from build123d import *

# Parameters (mm, degrees)
BOSS_EXTRUDE1_DEPTH = 5.07492
SKETCH6_R           = 22.225
BOSS_EXTRUDE3_DEPTH = 5.07492
SKETCH2_3_R         = 6.35
CUT_EXTRUDE2_DEPTH  = 5.588
SKETCH8_W           = 2.728150378
SKETCH8_H           = 127
BOSS_EXTRUDE4_DEPTH = 5.07492
SKETCH9_W           = 1.905
SKETCH9_H           = 127
BOSS_EXTRUDE5_DEPTH = 5.07492
SKETCH12_R          = 3
CUT_EXTRUDE3_DEPTH  = 400.05
CUT_EXTRUDE4_START  = -5.07492
SKETCH13_R          = 22.86
SKETCH13_R_2        = 2
SKETCH13_R_3        = 6.35
CUT_EXTRUDE4_DEPTH  = 0.254
CUT_EXTRUDE6_START  = -127
SKETCH13_2_R        = 2
CUT_EXTRUDE6_DEPTH  = 127
SKETCH17_R          = 2.9972
CUT_EXTRUDE7_DEPTH  = 152.4
CUT_EXTRUDE8_START  = -1549.4
SKETCH13_3_R        = 6.35
CUT_EXTRUDE8_DEPTH  = 1549.4
SKETCH18_R          = 3.175
SKETCH18_R_2        = 2.159
SKETCH18_R_3        = 1.524
CUT_EXTRUDE9_DEPTH  = 6.35
SKETCH19_R          = 1.905
CUT_EXTRUDE10_DEPTH = 6.35


with BuildPart() as part:
    # Sketch2 → Boss-Extrude1 (new body)
    with BuildSketch(Plane.XY):
        with BuildLine():
            Line((-143.383, -31.75), (-127.127, -31.75))
            ThreePointArc((-127.127, -31.75), (-123.317, -30.48), (-119.507, -31.75))
            Line((-119.507, -31.75), (119.253, -31.75))
            ThreePointArc((119.253, -31.75), (123.063, -30.48), (126.873, -31.75))
            Line((126.873, -31.75), (143.383, -31.75))
            Line((143.383, -31.75), (143.383, 95.25))
            Line((143.383, 95.25), (-143.383, 95.25))
            Line((-143.383, 95.25), (-143.383, -31.75))
        make_face()
    extrude(amount=-BOSS_EXTRUDE1_DEPTH)

    # Sketch6 → Boss-Extrude3 (add)
    with BuildSketch(Plane(origin=(0, 0, -5.07492), x_dir=(-1, 0, 0), z_dir=(0, 0, -1))):
        with Locations((-123.063, -36.83)):
            Circle(SKETCH6_R)
        with Locations((123.317, -36.83)):
            Circle(SKETCH6_R)
    extrude(amount=-BOSS_EXTRUDE3_DEPTH)

    # Sketch2<3> → Cut-Extrude2 (cut)
    with BuildSketch(Plane.XY):
        with Locations((-123.317, -36.83)):
            Circle(SKETCH2_3_R)
        with Locations((123.063, -36.83)):
            Circle(SKETCH2_3_R)
    extrude(amount=-CUT_EXTRUDE2_DEPTH, mode=Mode.SUBTRACT)

    # Sketch8 → Boss-Extrude4 (add)
    with BuildSketch(Plane(origin=(0, 0, -5.07492), x_dir=(-1, 0, 0), z_dir=(0, 0, -1))):
        with Locations((144.139824811, 31.75)):
            Rectangle(SKETCH8_W, SKETCH8_H)
    extrude(amount=-BOSS_EXTRUDE4_DEPTH)

    # Sketch9 → Boss-Extrude5 (add)
    with BuildSketch(Plane(origin=(0, 0, -5.07492), x_dir=(-1, 0, 0), z_dir=(0, 0, -1))):
        with Locations((-144.3355, 31.75)):
            Rectangle(SKETCH9_W, SKETCH9_H)
    extrude(amount=-BOSS_EXTRUDE5_DEPTH)

    # Sketch12 → Cut-Extrude3 (cut)
    with BuildSketch(Plane.XY):
        with Locations((-123.317, 76.2)):
            Circle(SKETCH12_R)
        with Locations((123.063, 76.2)):
            Circle(SKETCH12_R)
    extrude(amount=-CUT_EXTRUDE3_DEPTH, mode=Mode.SUBTRACT)

    # Sketch13 → Cut-Extrude4 (cut)
    # profile 1 of 2: a face of its own
    with BuildSketch(Plane(origin=(0, 0, -5.07492), x_dir=(-1, 0, 0), z_dir=(0, 0, -1)).offset(CUT_EXTRUDE4_START)):
        with Locations(Location((23.352511843, 49.53, 0), (0, 0, 180))):
            Circle(SKETCH13_R)
        with Locations(Location((23.352511843, 67.0306, 0), (0, 0, 180))):
            Circle(SKETCH13_R_2, mode=Mode.SUBTRACT)
        with Locations(Location((40.853111843, 49.53, 0), (0, 0, 180))):
            Circle(SKETCH13_R_2, mode=Mode.SUBTRACT)
        with Locations(Location((23.352511843, 32.0294, 0), (0, 0, 180))):
            Circle(SKETCH13_R_2, mode=Mode.SUBTRACT)
        with Locations(Location((5.851911843, 49.53, 0), (0, 0, 180))):
            Circle(SKETCH13_R_2, mode=Mode.SUBTRACT)
        with Locations(Location((23.352511843, 49.53, 0), (0, 0, 180))):
            Circle(SKETCH13_R_3, mode=Mode.SUBTRACT)
    # profile 2 of 2: a face of its own
    with BuildSketch(Plane(origin=(0, 0, -5.07492), x_dir=(-1, 0, 0), z_dir=(0, 0, -1)).offset(CUT_EXTRUDE4_START)):
        with Locations(Location((-32.2961, 1.27, 0), (0, 0, 180))):
            Circle(SKETCH13_R)
        with Locations(Location((-32.2961, 18.7706, 0), (0, 0, 180))):
            Circle(SKETCH13_R_2, mode=Mode.SUBTRACT)
        with Locations(Location((-14.7955, 1.27, 0), (0, 0, 180))):
            Circle(SKETCH13_R_2, mode=Mode.SUBTRACT)
        with Locations(Location((-32.2961, -16.2306, 0), (0, 0, 180))):
            Circle(SKETCH13_R_2, mode=Mode.SUBTRACT)
        with Locations(Location((-49.7967, 1.27, 0), (0, 0, 180))):
            Circle(SKETCH13_R_2, mode=Mode.SUBTRACT)
        with Locations(Location((-32.2961, 1.27, 0), (0, 0, 180))):
            Circle(SKETCH13_R_3, mode=Mode.SUBTRACT)
    extrude(amount=CUT_EXTRUDE4_DEPTH, mode=Mode.SUBTRACT)

    # Sketch13<2> → Cut-Extrude6 (cut)
    with BuildSketch(Plane(origin=(0, 0, -5.07492), x_dir=(-1, 0, 0), z_dir=(0, 0, -1)).offset(CUT_EXTRUDE6_START)):
        with Locations((-32.2961, 18.7706)):
            Circle(SKETCH13_2_R)
        with Locations((-49.7967, 1.27)):
            Circle(SKETCH13_2_R)
        with Locations((-14.7955, 1.27)):
            Circle(SKETCH13_2_R)
        with Locations((-32.2961, -16.2306)):
            Circle(SKETCH13_2_R)
        with Locations((23.352511843, 32.0294)):
            Circle(SKETCH13_2_R)
        with Locations((23.352511843, 67.0306)):
            Circle(SKETCH13_2_R)
        with Locations((40.853111843, 49.53)):
            Circle(SKETCH13_2_R)
        with Locations((5.851911843, 49.53)):
            Circle(SKETCH13_2_R)
    extrude(amount=CUT_EXTRUDE6_DEPTH, mode=Mode.SUBTRACT)

    # Sketch17 → Cut-Extrude7 (cut)
    with BuildSketch(Plane(origin=(0, 0, -5.07492), x_dir=(-1, 0, 0), z_dir=(0, 0, -1))):
        with Locations((87.0839, -19.05)):
            Circle(SKETCH17_R)
        with Locations((-86.868, -16.51)):
            Circle(SKETCH17_R)
    extrude(amount=-CUT_EXTRUDE7_DEPTH, mode=Mode.SUBTRACT)

    # Sketch13<3> → Cut-Extrude8 (cut)
    with BuildSketch(Plane(origin=(0, 0, -5.07492), x_dir=(-1, 0, 0), z_dir=(0, 0, -1)).offset(CUT_EXTRUDE8_START)):
        with Locations((-32.2961, 1.27)):
            Circle(SKETCH13_3_R)
        with Locations((23.352511843, 49.53)):
            Circle(SKETCH13_3_R)
    extrude(amount=CUT_EXTRUDE8_DEPTH, mode=Mode.SUBTRACT)

    # Sketch18 → Cut-Extrude9 (cut)
    with BuildSketch(Plane(origin=(0, 0, -5.07492), x_dir=(-1, 0, 0), z_dir=(0, 0, -1))):
        with Locations((14.5669, -22.225)):
            Circle(SKETCH18_R)
        with Locations((-68.691950102, 24.511)):
            Circle(SKETCH18_R_2)
        with Locations((-62.682085042, -3.620822534)):
            Circle(SKETCH18_R_3)
        with Locations((-1.953743286, -3.620822534)):
            Circle(SKETCH18_R_3)
        with Locations((-12.06825034, -21.868989912)):
            Circle(SKETCH18_R_3)
        with Locations((-52.96225034, -21.321575615)):
            Circle(SKETCH18_R_3)
        with Locations((-6.972782316, 44.115913262)):
            Circle(SKETCH18_R_3)
        with Locations((2.749026104, 26.629515804)):
            Circle(SKETCH18_R_3)
        with Locations((43.955997581, 26.629515804)):
            Circle(SKETCH18_R_3)
        with Locations((53.677806001, 44.115913262)):
            Circle(SKETCH18_R_3)
    extrude(amount=-CUT_EXTRUDE9_DEPTH, mode=Mode.SUBTRACT)

    # Sketch19 → Cut-Extrude10 (cut)
    with BuildSketch(Plane(origin=(0, 0, -5.07492), x_dir=(-1, 0, 0), z_dir=(0, 0, -1))):
        with Locations((-130.937, -20.884382673)):
            Circle(SKETCH19_R)
        with Locations((-114.458147951, -20.884382673)):
            Circle(SKETCH19_R)
        with Locations((-123.063, -48.133)):
            Circle(SKETCH19_R)
        with Locations((115.501615385, -20.779600443)):
            Circle(SKETCH19_R)
        with Locations((132.011615385, -20.779600443)):
            Circle(SKETCH19_R)
        with Locations((123.317, -48.133)):
            Circle(SKETCH19_R)
    extrude(amount=-CUT_EXTRUDE10_DEPTH, mode=Mode.SUBTRACT)


solid = part.part
Design review of the part built by this model. Coordinates are the model's own, in mm. A direction names the side the tool comes from. Give positions to 0.01 mm unless a question says otherwise; leave off trailing zeros. Loops run counter-clockwise (first coordinate to the right, second up) from the corner with the lowest first, then second, coordinate; pieces in that order, holes last. Notation, with made-up numbers: (-39, 43.25) - (-4, 43.25) arc R28 ccw to (-4, 74.25) - close; hole circle Ø4 at (-11.75, 69.5). An arc over 180 degrees is marked (long way). Write item = value, one per line.
1) Clearance check with flat-ended pins moving along their axes: pin 1 Ø3 at (x, y) = (-115.5, -20.78) entering from +Z; pin 2 Ø4 at (x, y) = (-28, 50.5) entering from +Z. State where each tip first meets the part, or that it passes through.
Result sheet:
pin_1 = through
pin_2 = -0.25
2) Take a section at C-C on x = 74.5. State the section outline as (y, z) points, and give its area (3 significant figures).
Result sheet:
outline = (-31.75, -5.07) - (95.25, -5.07) - (95.25, 0) - (-31.75, 0) - close
area = 645 mm2
3) Take a section at B-B on y = 76.2. State the section outline as (x, z) points, and give its area (3 significant figures).
Result sheet:
outline = (-145.5, -5.07) - (-126.32, -5.07) - (-126.32, 0) - (-145.5, 0) - close; (-120.32, -5.07) - (120.06, -5.07) - (120.06, 0) - (-120.32, 0) - close; (126.06, -5.07) - (145.29, -5.07) - (145.29, 0) - (126.06, 0) - close
area = 1,410 mm2
4) To check wall thickness, follow line 1 (X direction, y = 1.27, z = -3.05); line 2 (X direction, y = 50, z = -4.65); line 3 (Y direction, x = -15, z = -3.3). State the ranges of each line that lie inside material, in increasing order.
Result sheet:
line_1 = -145.5 to 12.8, 16.8 to 25.95, 38.65 to 47.8, 51.8 to 145.29
line_2 = -145.5 to -42.8, -38.91 to -29.69, -17.02 to -7.8, -3.91 to 145.29
line_3 = -31.75 to -25.37, -19.08 to 95.25
5) Tool access review of faces 1 (the face through (85.26, -13.98, -2.57)), 2 (the face through (37, 6, -0.254)): name each direction out of +Z, -Z, +X, -X, +Y, -Y from which nothing blocks a thin tool from reaching the whole face with its end or side.
Result sheet:
face_1 = +Z, -Z
face_2 = +Z
6) Take a section at A-A on y = -36.83. State the section outline as (x, z) points.
Result sheet:
outline = (-145.54, -5.07) - (-129.67, -5.07) - (-129.67, 0) - (-145.54, 0) - close; (-116.97, -5.07) - (-101.09, -5.07) - (-101.09, 0) - (-116.97, 0) - close; (100.84, -5.07) - (116.71, -5.07) - (116.71, 0) - (100.84, 0) - close; (129.41, -5.07) - (145.29, -5.07) - (145.29, 0) - (129.41, 0) - close
7) Take a section at D-D on z = -3.4. Count the separate pieces of the cut face and the enclosed holes in it, and give its area (3 significant figures).
Result sheet:
separate_pieces = 1
enclosed_holes = 32
area = 38,000 mm2
8) Draft analysis for pull direction Y (two halves, no side actions). For faces 3 (the face through (2, 95.25, -3)), 4 (the face through (2, 36, -5.075)), 5 (the face through (-14.154, -19.077, -2.573)), state which applies: +Y half, -Y half, draft (parallel to the pull), parting line (faces both ways), or undercut.
Result sheet:
face_3 = +Y half
face_4 = draft
face_5 = undercut
